from build123d import *

# Parameters (mm, degrees)
SKETCH_1_R          = 5
EXTRUDE_1_DEPTH     = 3
SKETCH_2_W          = 3
SKETCH_2_H          = 10
SKETCH_2_W_2        = 10
SKETCH_2_H_2        = 3
CUT_EXTRUDE_1_DEPTH = 225.320807502


with BuildPart() as part:
    # 草图1 → 凸台-拉伸1 (new body)
    # profile 1 of 2: a face of its own
    with BuildSketch(Plane(origin=(0, 0, 0), x_dir=(1, 0, 0), z_dir=(0, 1, 0))):
        with BuildLine():
            Line((-189.5, 2.67807522), (-189.5, -2.67807522))
            add(Edge.make_bspline(
                [(-189.5, -2.67807522), (-189.403013737, -5.4287659), (-188.913529521, -11.280436832), (-187.184797767, -20.477000703), (-182.901604371, -32.558534689), (-176.518140993, -44.473382271), (-168.370672682, -55.661029172), (-158.816512899, -65.937496211), (-145.622389947, -77.408485785), (-128.233359888, -89.122185343), (-106.405311843, -100.093014988), (-80.328404186, -109.345622083), (-53.415456511, -115.716654886), (-26.01245021, -119.406694681), (1.612249886, -120.52669773), (29.223526803, -119.1102282), (56.584216313, -115.114894197), (83.419619157, -108.420073225), (109.201033267, -98.876697436), (130.527468144, -87.756954706), (147.425203381, -76.001107817), (160.172847856, -64.598888808), (169.450747209, -54.337956503), (177.420154922, -43.019542435), (183.422267467, -31.306804293), (187.385215446, -19.571139093), (188.958191111, -10.7853005), (189.405454524, -5.359541143), (189.5, -2.67807522)],
                knots=[0, 0, 0, 0, 0, 0.022605252, 0.048189512, 0.076525509, 0.104866865, 0.133209133, 0.161552255, 0.191528088, 0.248214577, 0.304901251, 0.361587924, 0.418274582, 0.474961249, 0.531647919, 0.588334591, 0.645021247, 0.701707888, 0.758394507, 0.813600526, 0.841943986, 0.87028688, 0.898629863, 0.926970611, 0.955317967, 0.977963639, 1, 1, 1, 1, 1], degree=4))
            Line((189.5, -2.67807522), (189.5, 2.67807522))
            add(Edge.make_bspline(
                [(-189.5, 2.67807522), (-189.403013737, 5.4287659), (-188.913529521, 11.280436832), (-187.184797767, 20.477000703), (-182.901604371, 32.558534689), (-176.518140993, 44.473382271), (-168.370672682, 55.661029172), (-158.816512899, 65.937496211), (-145.622389947, 77.408485785), (-128.233359888, 89.122185343), (-106.405311843, 100.093014988), (-80.328404186, 109.345622083), (-53.415456511, 115.716654886), (-26.01245021, 119.406694681), (1.612249886, 120.52669773), (29.223526803, 119.1102282), (56.584216313, 115.114894197), (83.419619157, 108.420073225), (109.201033267, 98.876697436), (130.527468144, 87.756954706), (147.425203381, 76.001107817), (160.172847856, 64.598888808), (169.450747209, 54.337956503), (177.420154922, 43.019542435), (183.422267467, 31.306804293), (187.385215446, 19.571139093), (188.958191111, 10.7853005), (189.405454524, 5.359541143), (189.5, 2.67807522)],
                knots=[0, 0, 0, 0, 0, 0.022605252, 0.048189512, 0.076525509, 0.104866865, 0.133209133, 0.161552255, 0.191528088, 0.248214577, 0.304901251, 0.361587924, 0.418274582, 0.474961249, 0.531647919, 0.588334591, 0.645021247, 0.701707888, 0.758394507, 0.813600526, 0.841943986, 0.87028688, 0.898629863, 0.926970611, 0.955317967, 0.977963639, 1, 1, 1, 1, 1], degree=4))
        make_face()
        with BuildLine():
            Line((159.5, 2.083418932), (159.5, -2.083418932))
            add(Edge.make_bspline(
                [(159.5, -2.083418932), (159.430377933, -3.619846345), (159.139385215, -6.671456978), (157.940786615, -12.816015531), (155.280316673, -20.500519912), (150.2464343, -29.63014035), (141.267593425, -41.375851732), (126.3637498, -54.741405415), (104.515298354, -67.83687478), (80.138153839, -77.866087876), (54.182309112, -84.909390201), (27.304092868, -89.081582998), (-2.6913e-05, -90.462801356), (-27.304083634, -89.081576827), (-54.182312778, -84.909404424), (-80.138151247, -77.866066645), (-104.515130919, -67.836936962), (-126.363664513, -54.74153076), (-141.267763099, -41.375581268), (-150.246208112, -29.630491802), (-155.280421928, -20.500291974), (-157.940686294, -12.816236482), (-159.139431477, -6.671261076), (-159.43038084, -3.619814978), (-159.5, -2.083423638)],
                knots=[0.001568685, 0.001568685, 0.001568685, 0.001568685, 0.017144663, 0.03272064, 0.063872596, 0.095024552, 0.126176507, 0.188480419, 0.25078433, 0.313088241, 0.375392153, 0.437696064, 0.499999976, 0.562303887, 0.624607798, 0.68691171, 0.749215621, 0.811519532, 0.873823444, 0.904975399, 0.936127355, 0.967279311, 0.982855289, 0.998431266, 0.998431266, 0.998431266, 0.998431266], degree=3))
            Line((-159.5, -2.083423638), (-159.5, 2.083423638))
            add(Edge.make_bspline(
                [(-159.5, 2.083423638), (-159.43038084, 3.619814978), (-159.139431477, 6.671261076), (-157.940686294, 12.816236482), (-155.280421928, 20.500291974), (-150.246208112, 29.630491802), (-141.267763099, 41.375581268), (-126.363664513, 54.74153076), (-104.515130919, 67.836936962), (-80.138151247, 77.866066645), (-54.182312778, 84.909404424), (-27.304083634, 89.081576827), (-2.6913e-05, 90.462801356), (27.304092868, 89.081582998), (54.182309112, 84.909390201), (80.138153839, 77.866087876), (104.515298354, 67.83687478), (126.3637498, 54.741405415), (141.267593425, 41.375851732), (150.2464343, 29.63014035), (155.280316673, 20.500519912), (157.940786615, 12.816015531), (159.139385215, 6.671456978), (159.430377933, 3.619846345), (159.5, 2.083418932)],
                knots=[0.001568685, 0.001568685, 0.001568685, 0.001568685, 0.017144663, 0.03272064, 0.063872596, 0.095024552, 0.126176507, 0.188480419, 0.25078433, 0.313088241, 0.375392153, 0.437696064, 0.499999976, 0.562303887, 0.624607798, 0.68691171, 0.749215621, 0.811519532, 0.873823444, 0.904975399, 0.936127355, 0.967279311, 0.982855289, 0.998431266, 0.998431266, 0.998431266, 0.998431266], degree=3))
        make_face(mode=Mode.SUBTRACT)
    # profile 2 of 2: a face of its own
    with BuildSketch(Plane(origin=(0, 0, 0), x_dir=(1, 0, 0), z_dir=(0, 1, 0))):
        with BuildLine():
            Line((15, -89.584088933), (15, 89.584088933))
            add(Edge.make_bspline(
                [(-15, 89.584087357), (-10.007870789, 89.863221211), (-1.3117e-05, 90.141566253), (10.007857262, 89.863223114), (15, 89.584088933)],
                knots=[0.465745288, 0.465745288, 0.465745288, 0.465745288, 0.499999976, 0.534254707, 0.534254707, 0.534254707, 0.534254707], degree=3))
            Line((-15, 89.584087357), (-15, -89.584087357))
            add(Edge.make_bspline(
                [(15, -89.584088933), (10.007857262, -89.863223114), (-1.3117e-05, -90.141566253), (-10.007870789, -89.863221211), (-15, -89.584087357)],
                knots=[0.465745244, 0.465745244, 0.465745244, 0.465745244, 0.499999976, 0.534254663, 0.534254663, 0.534254663, 0.534254663], degree=3))
        make_face()
        with Locations(Location((0, 0, 0), (0, 0, 270))):
            Circle(SKETCH_1_R, mode=Mode.SUBTRACT)
    extrude(amount=EXTRUDE_1_DEPTH)

    # 草图2 → 切除-拉伸1 (cut, through all)
    with BuildSketch(Plane(origin=(0, 3, 0), x_dir=(1, 0, 0), z_dir=(0, 1, 0))):
        with Locations((140, -65.874036058)):
            Rectangle(SKETCH_2_W, SKETCH_2_H)
        with Locations((174.473517333, -0.002394208)):
            Rectangle(SKETCH_2_W_2, SKETCH_2_H_2)
        with Locations((140, 65.869247642)):
            Rectangle(SKETCH_2_W, SKETCH_2_H)
        with Locations((70, -96.514031923)):
            Rectangle(SKETCH_2_W, SKETCH_2_H)
        with Locations((70, 96.509243508)):
            Rectangle(SKETCH_2_W, SKETCH_2_H)
        with Locations((0, 99.519533663)):
            Rectangle(SKETCH_2_W, SKETCH_2_H)
        with Locations((0, -99.524322078)):
            Rectangle(SKETCH_2_W, SKETCH_2_H)
        with Locations((-70, -96.514031923)):
            Rectangle(SKETCH_2_W, SKETCH_2_H)
        with Locations((-140, -65.874036058)):
            Rectangle(SKETCH_2_W, SKETCH_2_H)
        with Locations((-174.473517333, -0.002394208)):
            Rectangle(SKETCH_2_W_2, SKETCH_2_H_2)
        with Locations((-140, 65.869247642)):
            Rectangle(SKETCH_2_W, SKETCH_2_H)
        with Locations((-70, 96.509243508)):
            Rectangle(SKETCH_2_W, SKETCH_2_H)
    extrude(amount=-CUT_EXTRUDE_1_DEPTH, mode=Mode.SUBTRACT)


solid = part.part
Model file for the job. Use its own axes, mm. Coordinates: 2 decimals unless noted, no trailing zeros. Write each question's results on one line, items separated by ' | '. Start each with the question number.
1) Flat gauge pins, fed straight in: P1, Ø0.9, axis at x = -172, y = 2, coming from the -Z side; P2, Ø0.9, axis at y = 1.5, z = 15, coming from the -X side; P3, Ø1.5, axis at y = 1.5, z = 100.5, coming from the -X side. Where does each tip first touch, or does it go through?
2) Mould opens along Z. For faces 1 (the face through (-3, 0, 25)), 2 (the face through (-4.88, 1.48, -1.08)) say: pulls with the +Z half, pulls with the -Z half, needs draft (parallel to the pull), parting line crosses it, or undercut.
3) Cut at A-A (y = 0.55). Count the separate pieces of the cut face and the enclosed holes in it, then the cut area to 3 significant figures.
4) Probe line 1 along X through (y, z) = (1.55, 0); line 2 along X through (y, z) = (0.1, 92.5); line 3 along X through (y, z) = (1.15, 97). List the from-to ranges inside material, lowest first. Write a range as from..to.
Returned:
1) P1: z = -51.04 | P2: x = -188.15 | P3: x = -105.37
2) face 1: needs draft | face 2: undercut
3) separate pieces: 1 | enclosed holes: 15 | area: 31,700 mm^2
4) line 1: -189.5..-179.47, -169.47..-159.5, -15..-5, 5..15, 159.5..169.47, 179.47..189.5 | line 2: -120.75..-71.5, -68.5..68.5, 71.5..120.75 | line 3: -111.6..-71.5, -68.5..-1.5, 1.5..68.5, 71.5..111.6
